Autodesk Inventor part; units mm, degrees
ref_plane "YZ Plane" through (0, 0, 0) normal (1, 0, 0) x (0, 1, 0)
ref_plane "XZ Plane" through (0, 0, 0) normal (0, 1, 0) x (-1, 0, 0)
ref_plane "XY Plane" through (0, 0, 0) normal (0, 0, 1) x (1, 0, 0)
sketch "Sketch1" plane through (0, 0, 0) normal (1, 0, 0) x (0, 1, 0)
  line L0 (44.4049, 39.363) -> (-19.0951, 39.363)
  line L1 (-19.0951, 39.363) -> (-19.0951, -63.507)
  line L2 (-19.0951, -63.507) -> (44.4049, -63.507)
  line L3 (44.4049, -63.507) -> (44.4049, 39.363)
  point P0 (0, 0)
  dimension "d0" = 102.87
  dimension "d1" = 63.5
extrude "Extrusion1" add sketch "Sketch1" along normal blind 5.08
sketch "Sketch2" plane through (5.08, 0, 0) normal (1, 0, 0) x (0, 0, -1)
  line L0 (63.507, 44.4049) -> (-39.363, 44.4049)
  line L1 (-39.363, 44.4049) -> (-39.363, -19.0951)
  point P0 (0, 0)
  point P1 (-34.283, 39.3249)
  point P2 (54.617, 39.3249)
  point P3 (54.617, -8.3001)
  point P4 (-34.283, -8.3001)
  dimension "d4" = 0
  dimension "d5" = 0
  dimension "d6" = 0
  dimension "d7" = 0
  dimension "d8" = 88.9
  dimension "d9" = 5.08
  dimension "d10" = 5.08
  dimension "d11" = 47.625
hole "Hole1" at (5.08, 39.3249, 34.283) at (5.08, 39.3249, -54.617) at (5.08, -8.3001, -54.617) at (5.08, -8.3001, 34.283) direction (-1, 0, 0) diameter 5.1054 end through all
sketch "Sketch3" plane through (0, -19.0951, -63.507) normal (0, -1, 0) x (1, 0, 0)
  line L0 (-45.72, 0) -> (5.08, 0)
  line L1 (5.08, 0) -> (5.08, 102.87)
  line L2 (5.08, 102.87) -> (-45.72, 102.87)
  line L3 (-45.72, 102.87) -> (-45.72, 0)
  line L4 (5.08, 102.87) -> (5.08, 0)
  line L5 (0, 0) -> (5.08, 0)
  line L6 (0, 102.87) -> (5.08, 102.87)
  point P0 (0, 63.507)
  dimension "d19" = 0
  dimension "d20" = 0
  dimension "d21" = 0
  dimension "d22" = 50.8
extrude "Extrusion2" add sketch "Sketch3" along normal blind 5.08
sketch "Sketch4" plane through (0, -19.0951, -63.507) normal (0, 1, 0) x (1, 0, 0)
  line L0 (0, -102.87) -> (-45.72, -102.87)
  line L1 (-45.72, 0) -> (0, 0)
  line L2 (5.08, 0) -> (5.08, -102.87)
  point P0 (0, -63.507)
  point P1 (-7.62, -77.47)
  point P2 (-33.02, -77.47)
  point P3 (-33.02, -26.67)
  point P4 (-7.62, -26.67)
  dimension "d25" = 0
  dimension "d26" = 0
  dimension "d27" = 0
  dimension "d28" = 0
  dimension "d29" = 25.4
  dimension "d30" = 50.8
  dimension "d31" = 25.4
  dimension "d32" = 26.67
  dimension "d33" = 12.7
hole "Hole2" at (-7.62, -19.0951, 13.963) at (-33.02, -19.0951, 13.963) at (-33.02, -19.0951, -36.837) at (-7.62, -19.0951, -36.837) direction (0, -1, 0) diameter 5.1054 end through all
sketch "Sketch5" plane through (0, -24.1751, -63.507) normal (0, -1, 0) x (1, 0, 0)
  line L0 (-91.5665, 115.4463) -> (-40.64, 115.4463)
  line L1 (-40.64, 115.4463) -> (-40.64, -11.0997)
  line L2 (-40.64, -11.0997) -> (-91.5665, -11.0997)
  line L3 (-91.5665, -11.0997) -> (-91.5665, 115.4463)
  line L4 (-45.72, 102.87) -> (-45.72, 0)
  point P0 (0, 63.507)
  dimension "d41" = 5.08
extrude "Extrusion3" cut sketch "Sketch5" against normal blind 25.4
fillet "Fillet1" radius 6.35 4 edges at (-40.64, -21.6351, -63.507) (-40.64, -21.6351, 39.363) (2.54, 44.4049, 39.363) (2.54, 44.4049, -63.507)
properties part number "LimeLight90"
Could you check a few things on this model? Use its own coordinates, in mm. A direction names the side the tool comes from. Coordinates: 2 decimals unless noted, no trailing zeros. Order: outer loops, then holes, each group sorted by start corner. A loop starts at its lowest first (then second) coordinate and runs counter-clockwise, first axis right, second up. Notation, with made-up numbers: (70, -40) -> (94, -40) arc R13 ccw to (94, -24) -> close; hole circle Ø4 at (42.5, 62). An arc over 180 degrees is marked (long way). One line per question, with ' | ' between items.
Q1. On a 3-axis mill with a long thin cutter (end or side, diameter ignored), from which of +Z, -Z, +X, -X, +Y, -Y can I reach the whole of each face in a straight line? I mean faces 4 (the face through (-21, -19.095, -11)), 5 (the face through (2.504, 41.817, -54.064)). Say none if no direction works.
Return value:
face 4: +Z, -Z, -X, +Y | face 5: +X, -X
Q2. If I drill on L1, parallel to Z at x = -33.02, y = -20.4; L2, parallel to Y at x = -2, z = -3; L3, parallel to X at y = -4.5, z = 9.5, over which ranges is the centre line in solid material (lowest first)?
Return value:
L1: -63.51 to -39.39, -34.28 to 11.41, 16.52 to 39.36 | L2: -24.18 to -19.1 | L3: 0 to 5.08
Q3. I'm going to push flat-ended pins straight in: P1, Ø12, axis at x = -29.5, z = -12.5, coming from the +Y side; P2, Ø5, axis at y = 31.5, z = -23, coming from the -X side. Where does each tip first touch, or does it pass through?
Return value:
P1: y = -19.1 | P2: x = 0
Q4. Imagine slicing it at C-C on z = -54. Please give me the cut outline in (x, y).
Return value:
outline: (-40.64, -24.18) -> (5.08, -24.18) -> (5.08, -10.78) -> (0, -10.78) -> (0, -19.1) -> (-40.64, -19.1) -> close; (0, -5.82) -> (5.08, -5.82) -> (5.08, 36.85) -> (0, 36.85) -> close; (0, 41.8) -> (5.08, 41.8) -> (5.08, 44.4) -> (0, 44.4) -> close
Q5. Imagine slicing it at B-B on z = -36.5. Please give me the cut outline in (x, y), and give its area (3 significant figures).
Return value:
outline: (-40.64, -24.18) -> (-35.55, -24.18) -> (-35.55, -19.1) -> (-40.64, -19.1) -> close; (-30.49, -24.18) -> (-10.15, -24.18) -> (-10.15, -19.1) -> (-30.49, -19.1) -> close; (-5.09, -24.18) -> (5.08, -24.18) -> (5.08, 44.4) -> (0, 44.4) -> (0, -19.1) -> (-5.09, -19.1) -> close | area: 503 mm²
Q6. Imagine slicing it at D-D on x = -14. Please give me the cut outline in (y, z), and give its area (3 significant figures).
Return value:
outline: (-24.18, -63.51) -> (-19.1, -63.51) -> (-19.1, 39.36) -> (-24.18, 39.36) -> close | area: 523 mm²
Q7. Thinking about a two-plate mould opening in X: for faces 1 (the face through (2, -2, 39.363)), 2 (the face through (0, 12, -11)), 3 (the face through (-8.387, -21.671, -34.402)), which applies, pulls with the +X half, pulls with the -X half, needs draft (parallel to the pull), parting line crosses it, or undercut?
Return value:
face 1: needs draft | face 2: pulls with the -X half | face 3: undercut
Q8. Imagine slicing it at A-A on x = -33.02. Please give me the cut outline in (y, z).
Return value:
outline: (-24.18, -63.51) -> (-19.1, -63.51) -> (-19.1, -39.39) -> (-24.18, -39.39) -> close; (-24.18, -34.28) -> (-19.1, -34.28) -> (-19.1, 11.41) -> (-24.18, 11.41) -> close; (-24.18, 16.52) -> (-19.1, 16.52) -> (-19.1, 39.36) -> (-24.18, 39.36) -> close
